Build history of the part. All positions in model axes, mm. A direction names the side the tool comes from. Round coordinates to 2 decimals unless told otherwise and drop trailing zeros. Write each loop counter-clockwise with the first axis right and the second up, starting at its lowest first coordinate (ties: lowest second). Pieces come first, ordered by that corner, then holes. Notation, with made-up numbers: M 32.5,2 L 56.5,2 A21 cw 56.5,7 Z; hole C -28.75,52 d1. An arc over 180 degrees is marked long. Write item = value, one per line.
from build123d import *

# Parameters (mm, degrees)
SKETCH_1_R      = 5
EXTRUDE_1_DEPTH = 4


with BuildPart() as part:
    # Эскиз1 → Бобышка-Вытянуть1 (new body)
    with BuildSketch(Plane.XY):
        with BuildLine():
            Line((31.5, 0), (31.5, -4))
            Line((31.5, -4), (51.5, -4))
            Line((51.5, -4), (51.5, 0))
            Line((51.5, 0), (71.5, 0))
            Line((71.5, 0), (71.5, -4))
            Line((71.5, -4), (91.5, -4))
            Line((91.5, -4), (91.5, 0))
            Line((91.5, 0), (123, 0))
            Line((123, 0), (123, 20))
            Line((123, 20), (119, 20))
            Line((119, 20), (119, 40))
            Line((119, 40), (123, 40))
            Line((123, 40), (123, 60))
            Line((123, 60), (119, 60))
            Line((119, 60), (119, 80))
            Line((119, 80), (123, 80))
            Line((123, 80), (123, 100))
            Line((123, 100), (119, 100))
            Line((119, 100), (119, 120))
            Line((119, 120), (123, 120))
            Line((123, 120), (123, 144.5))
            ThreePointArc((123, 144.5), (114, 153.5), (105, 144.5))
            Line((105, 144.5), (105, 142))
            Line((105, 142), (0, 142))
            Line((0, 142), (0, 120))
            Line((0, 120), (4, 120))
            Line((4, 120), (4, 100))
            Line((4, 100), (0, 100))
            Line((0, 100), (0, 80))
            Line((0, 80), (4, 80))
            Line((4, 80), (4, 60))
            Line((4, 60), (0, 60))
            Line((0, 60), (0, 40))
            Line((0, 40), (4, 40))
            Line((4, 40), (4, 20))
            Line((4, 20), (0, 20))
            Line((0, 20), (0, 0))
            Line((0, 0), (31.5, 0))
        make_face()
        with Locations((114, 144.5)):
            Circle(SKETCH_1_R, mode=Mode.SUBTRACT)
    extrude(amount=EXTRUDE_1_DEPTH)


solid = part.part
1. Mould opens along Y. For faces 1 (the face through (121, 40, 2)), 2 (the face through (0, 50, 2)), 3 (the face through (16, 0, 2)) say: pulls with the +Y half, pulls with the -Y half, needs draft (parallel to the pull), parting line crosses it, or undercut.
Responses:
face_1 = undercut
face_2 = needs draft
face_3 = pulls with the -Y half
2. Band-saw the part on B-B (x = 61.5). List the corners of the cut face in (y, z).
Responses:
outline = M 0,0 L 142,0 L 142,4 L 0,4 Z
3. Flat gauge pins, fed straight in: pin 1 (2 mm diameter, centred on y = -2, z = 1.5, fed in from -X); pin 2 (1.2 mm diameter, centred on x = 121.5, z = 1.5, fed in from -Y); pin 3 (1.2 mm diameter, centred on x = 75.5, z = 2, fed in from +Y). Where does each tip first touch, or does it go through?
Responses:
pin_1 = 31.5
pin_2 = 0
pin_3 = 142
4. Band-saw the part on A-A (x = 114). List the corners of the cut face in (y, z).
Responses:
outline = M 0,0 L 139.5,0 L 139.5,4 L 0,4 Z; M 149.5,0 L 153.5,0 L 153.5,4 L 149.5,4 Z
5. Band-saw the part on C-C (y = 30). List the corners of the cut face in (x, z).
Responses:
outline = M 4,0 L 119,0 L 119,4 L 4,4 Z
6. Probe probe 1 along Y at (x, z) = (15, 1.85); probe 2 along Y at (x, z) = (114, 0.95); probe 3 along Y at (x, z) = (33.5, 2). List the from-to ranges inside material, lowest first.
Responses:
probe_1 = 0 to 142
probe_2 = 0 to 139.5, 149.5 to 153.5
probe_3 = -4 to 142
7. Tool access for faces 4 (the face through (107, 0, 2)), 5 (the face through (121, 120, 2)), 6 (the face through (51.5, -2, 2)), 7 (the face through (4, 70, 2)): list every direction of +Z, -Z, +X, -X, +Y, -Y with a clear straight run to the whole face (end or side of a thin tool).
Responses:
face_4 = +Z, -Z, +X, -Y
face_5 = +Z, -Z, +X
face_6 = +Z, -Z, -Y
face_7 = +Z, -Z, -X
